Verification items for the finished model (mm, model axes). Coordinates: 2 decimals unless noted, no trailing zeros. Order: outer loops, then holes, each group sorted by start corner. A loop starts at its lowest first (then second) coordinate and runs counter-clockwise, first axis right, second up. Notation, with made-up numbers: (44, 21) -> (96, 21) arc R23 ccw to (96, 47) -> close; hole circle Ø9 at (47, 2). An arc over 180 degrees is marked (long way). Write each question's results on one line, items separated by ' | '. Start each with the question number.
(1) Thickness scan on probe 1 along X at (y, z) = (399.5, 11.5); probe 2 along X at (y, z) = (444.5, 3.25); probe 3 along Y at (x, z) = (43.5, 6.5). Record the ranges inside material, lowest first. Write a range as [from, to].
(2) Go/stop test with flat-tipped pins: pin 1 (3 mm diameter, centred on y = 581, z = 4.5, fed in from -X); pin 2 (1 mm diameter, centred on y = 566, z = 5, fed in from +X); pin 3 (6 mm diameter, centred on y = 444.5, z = 7, fed in from +X). Record where each tip stops, or that it passes through.
(3) Cross-section at C-C on z = 5.25. Enter the section's corners in (x, y), and give its area (3 significant figures).
```python
from build123d import *

# Parameters (mm, degrees)
SKETCH1_W           = 500
SKETCH1_H           = 800
BOSS_EXTRUDE1_DEPTH = 12
SKETCH1_5_W         = 452
SKETCH1_5_H         = 276
CUT_EXTRUDE1_DEPTH  = 944.474429966
CHAMFER1_SIZE       = 12


with BuildPart() as part:
    # Sketch1 → Boss-Extrude1 (new body)
    with BuildSketch(Plane.XY):
        with Locations((250, 400)):
            Rectangle(SKETCH1_W, SKETCH1_H)
    extrude(amount=BOSS_EXTRUDE1_DEPTH)

    # Sketch1<5> → Cut-Extrude1 (cut, through all)
    with BuildSketch(Plane.XY):
        with Locations((250, 400)):
            Rectangle(SKETCH1_5_W, SKETCH1_5_H)
    extrude(amount=CUT_EXTRUDE1_DEPTH, mode=Mode.SUBTRACT)

    # Chamfer1
    chamfer1_edges = [part.edges().sort_by_distance(p)[0] for p in [
        (250, 0, 0),
        (0, 400, 0),
        (250, 800, 0),
        (500, 400, 0),
    ]]
    chamfer(chamfer1_edges, length=CHAMFER1_SIZE - 0.0001)  # a hair under: the kernel refuses the full size


solid = part.part
```
Results are:
1) probe 1: x = [0.5, 24], [476, 499.5] | probe 2: x = [8.75, 24], [476, 491.25] | probe 3: y = [5.5, 262], [538, 794.5]
2) pin 1: stops at x = 6 | pin 2: stops at x = 493.5 | pin 3: stops at x = 498
3) outline: (6.75, 6.75) -> (493.25, 6.75) -> (493.25, 793.25) -> (6.75, 793.25) -> close; hole (24, 262) -> (476, 262) -> (476, 538) -> (24, 538) -> close | area: 258,000 mm2
